The listing builds one solid part. Answer for the finished solid, in the listing's coordinates (mm). Give positions to 0.01 mm unless a question says otherwise; leave off trailing zeros. Loops run counter-clockwise (first coordinate to the right, second up) from the corner with the lowest first, then second, coordinate; pieces in that order, holes last. Notation, with made-up numbers: (-8.75, 83.5) - (-2.75, 83.5) arc R33 cw to (-2.75, 114.5) - close; hole circle Ø10 at (71, 31). An arc over 180 degrees is marked (long way). Write item = value, one per line. Start each with the question number.
1) The part is cut by section A-A on y = 12.5. Write down the section's boundary in (x, z) (3 decimals).
2) Flat-ended cylindrical pins translate along their axes: P1, Ø9, axis at y = 9.525, z = 38.1, coming from the +X side; P2, Ø7, axis at x = 34.925, z = -34.925, coming from the -Y side; P3, Ø6, axis at y = 9.525, z = 38.1, coming from the -X side. Find the tip coordinate at first contact, or state that the pin passes through.
3) Consider probe 1 along X at (y, z) = (14.25, -35); probe 2 along Y at (x, z) = (92.75, -38.1) (3 decimals); probe 3 along X at (y, z) = (15.75, 36). Determine where each line is inside the solid, lowest interval first.
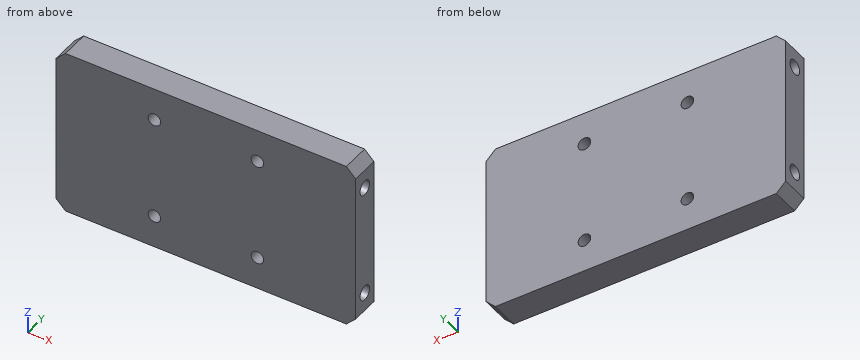
from build123d import *

# Parameters (mm, degrees)
SKETCH1_W              = 203.2
SKETCH1_H              = 114.3
BOSS_EXTRUDE1_DEPTH    = 19.05
SKETCH2_R              = 5
CUT_EXTRUDE1_DEPTH     = 19.05
CHAMFER1_SIZE          = 6.35
M10X1_5_TAPPED_HOLE1_D = 8.5


with BuildPart() as part:
    # Sketch1 → Boss-Extrude1 (new body)
    with BuildSketch(Plane(origin=(0, 0, 0), x_dir=(1, 0, 0), z_dir=(0, 1, 0))):
        Rectangle(SKETCH1_W, SKETCH1_H)
    extrude(amount=BOSS_EXTRUDE1_DEPTH)

    # Sketch2 → Cut-Extrude1 (cut)
    with BuildSketch(Plane.ZY.offset(101.6)):
        with Locations((-38.1, 9.525)):
            Circle(SKETCH2_R)
        with Locations((38.1, 9.525)):
            Circle(SKETCH2_R)
    cut_extrude1 = extrude(amount=-CUT_EXTRUDE1_DEPTH, mode=Mode.SUBTRACT)

    # Mirror1: Cut-Extrude1 across plane
    add(cut_extrude1.mirror(Plane(origin=(0, 0, 0), x_dir=(0, 0, 1), z_dir=(1, 0, 0))), mode=Mode.SUBTRACT)

    # Chamfer1
    chamfer1_edges = [part.edges().sort_by_distance(p)[0] for p in [
        (101.6, 9.525, 57.15),
        (-101.6, 9.525, 57.15),
        (-101.6, 9.525, -57.15),
        (101.6, 9.525, -57.15),
    ]]
    chamfer(chamfer1_edges, length=CHAMFER1_SIZE)

    # M10x1.5 Tapped Hole1 (through all)
    with Locations(Plane(origin=(0, 19.05, 0), x_dir=(1, 0, 0), z_dir=(0, 1, 0))):
        with Locations((34.925, -34.925), (-34.925, -34.925), (34.925, 34.925), (-34.925, 34.925)):
            Hole(M10X1_5_TAPPED_HOLE1_D / 2)


solid = part.part
Answer below:
q1.outline = (-101.6, -50.8) - (-95.25, -57.15) - (95.25, -57.15) - (101.6, -50.8) - (101.6, -42.119) - (82.55, -42.119) - (82.55, -34.081) - (101.6, -34.081) - (101.6, 34.081) - (82.55, 34.081) - (82.55, 42.119) - (101.6, 42.119) - (101.6, 50.8) - (95.25, 57.15) - (-95.25, 57.15) - (-101.6, 50.8) - (-101.6, 42.119) - (-82.55, 42.119) - (-82.55, 34.081) - (-101.6, 34.081) - (-101.6, -34.081) - (-82.55, -34.081) - (-82.55, -42.119) - (-101.6, -42.119) - close; hole circle Ø8.5 at (-34.925, -34.925); hole circle Ø8.5 at (-34.925, 34.925); hole circle Ø8.5 at (34.925, -34.925); hole circle Ø8.5 at (34.925, 34.925)
q2.P1 = 82.55
q2.P2 = through
q2.P3 = -82.55
q3.probe_1 = -101.6 to -39.17, -30.68 to 30.68, 39.17 to 101.6
q3.probe_2 = 0 to 4.525, 14.525 to 19.05
q3.probe_3 = -101.6 to -39.04, -30.81 to 30.81, 39.04 to 101.6
